Autodesk Inventor part; units mm, degrees
ref_plane "YZ Plane" through (0, 0, 0) normal (1, 0, 0) x (0, 1, 0)
ref_plane "XZ Plane" through (0, 0, 0) normal (0, 1, 0) x (-1, 0, 0)
ref_plane "XY Plane" through (0, 0, 0) normal (0, 0, 1) x (1, 0, 0)
sketch "Sketch1" plane through (0, 0, 0) normal (0, 1, 0) x (-1, 0, 0)
  line L0 (0, -15) -> (40, -15)
  line L1 (0, -54.7509) -> (0, -44.7509)
  line L2 (20, -23.5) -> (0, -23.5)
  line L3 (0, -23.5) -> (0, -15)
  circle A0 centre (5.2574, -19.75) radius 1.75
  line L4 (47.2, -27.5) -> (0, -54.7509)
  line L5 (0, -44.7509) -> (20, -33.2039)
  line L6 (20, -23.5) -> (20, -33.2039)
  line L7 (0, 15) -> (40, 15)
  line L8 (0, 54.7509) -> (0, 44.7509)
  line L9 (20, 23.5) -> (0, 23.5)
  line L10 (0, 23.5) -> (0, 15)
  circle A1 centre (5.2574, 19.75) radius 1.75
  line L11 (47.2, 27.5) -> (0, 54.7509)
  line L12 (0, 44.7509) -> (20, 33.2039)
  line L13 (20, 23.5) -> (20, 33.2039)
  line L14 (47.2, 27.5) -> (47.2, -27.5)
  line L15 (40, 15) -> (40, -15)
  line L16 (56.64, 0) -> (-9.44, 0)
  line L17 (0, -76.6513) -> (0, 76.6513)
  point P0 (0, 0)
  point P1 (0, 19.25)
  dimension "d3" = 15
  dimension "d6" = 5.2573
  dimension "d7" = 3.5
  dimension "d8" = 8.5
  dimension "d10" = 10
  dimension "d13" = 47.2
  dimension "d15" = 39.5
  dimension "d29" = 15
  dimension "d30" = 5.2573
  dimension "d31" = 40
  dimension "d32" = 19.75
  dimension "d33" = 8.5
  dimension "d34" = 20
  dimension "d35" = 20
  dimension "d37" = 60
  dimension "d38" = 60
  dimension "d39" = 55
  dimension "d40" = 27.5
  dimension "d41" = 10
  dimension "d68" = 21.2509
extrude "Extrusion1" add sketch "Sketch1" along normal blind 3 contours L0 L15 L16 L14 L4 L1 L5 L6 L2 L3 | L15 L7 L10 L9 L13 L12 L8 L11 L14 L16
sketch "Sketch2" plane through (0, 3, 0) normal (0, 1, 0) x (1, 0, 0)
  line L0 (-42.8964, 23) -> (-44.8964, 23)
  line L1 (-2.0164, 49.7415) -> (-1.0164, 48.0094)
  line L2 (-40.8535, 25.0094) -> (-41.8535, 26.7415)
  line L3 (-1.0164, -48.0094) -> (-2.0164, -49.7415)
  line L4 (-41.8535, -26.7415) -> (-40.8535, -25.0094)
  line L5 (-40.9205, -31.1255) -> (-39.2554, -28.2415)
  line L6 (-38.2554, -26.5094) -> (-36.5904, -23.6255)
  line L7 (-42.8964, -19.564) -> (-40.5928, -19.564)
  line L8 (-44.8964, -19.564) -> (-47.2, -19.564)
  line L9 (-47.2, 27.5) -> (-47.2, -27.5)
  line L10 (-47.2, -27.5) -> (-40.9205, -31.1255)
  line L11 (-47.2, -27.5) -> (0, -54.7509)
  line L12 (-4.6144, -48.2415) -> (-6.2795, -51.1255)
  line L13 (-3.6144, -46.5094) -> (-1.9494, -43.6255)
  line L14 (0, -44.7509) -> (-20, -33.2039)
  line L15 (-39.2554, 28.2415) -> (-40.9205, 31.1255)
  line L16 (-38.2554, 26.5094) -> (-36.5904, 23.6255)
  line L17 (-3.6144, 46.5094) -> (-1.9494, 43.6255)
  line L18 (-4.6144, 48.2415) -> (-6.2795, 51.1255)
  line L19 (-38.2554, -26.5094) -> (-40.8535, -25.0094)
  line L20 (-41.8535, -26.7415) -> (-39.2554, -28.2415)
  line L21 (-42.8964, -23) -> (-42.8964, -19.564)
  line L22 (-4.6144, -48.2415) -> (-2.0164, -49.7415)
  line L23 (-3.6144, -46.5094) -> (-1.0164, -48.0094)
  line L24 (-6.2795, -51.1255) -> (0, -54.7509)
  line L25 (0, -54.7509) -> (0, -44.7509)
  line L26 (0, -44.7509) -> (-1.9494, -43.6255)
  line L27 (-40.8535, 25.0094) -> (-38.2554, 26.5094)
  line L28 (-41.8535, 26.7415) -> (-39.2554, 28.2415)
  line L29 (-3.6144, 46.5094) -> (-1.0164, 48.0094)
  line L30 (-4.6144, 48.2415) -> (-2.0164, 49.7415)
  line L31 (-1.9494, 43.6255) -> (0, 44.7509)
  line L32 (0, 54.7509) -> (-6.2795, 51.1255)
  line L33 (0, 44.7509) -> (0, 54.7509)
  line L34 (-42.8964, 23) -> (-42.8964, 19.564)
  line L35 (-42.8964, 19.564) -> (-40.5928, 19.564)
  line L36 (-44.8964, 19.564) -> (-47.2, 19.564)
  line L37 (-47.2, 19.564) -> (-47.2, 27.5)
  line L38 (-47.2, 27.5) -> (-40.9205, 31.1255)
  line L39 (0, 54.7509) -> (-47.2, 27.5)
  line L40 (-20, 33.2039) -> (0, 44.7509)
  line L41 (-44.8964, -19.564) -> (-44.8964, -23)
  line L42 (-44.8964, -23) -> (-42.8964, -23)
  line L43 (-36.5904, 23.6255) -> (-40.5928, 21.3147)
  line L44 (-36.5904, -23.6255) -> (-40.5928, -21.3147)
  line L45 (-40.5928, -21.3147) -> (-40.5928, -19.564)
  line L46 (-40.5928, 19.564) -> (-40.5928, 21.3147)
  line L47 (-47.2, -27.5) -> (-47.2, -19.564)
  line L48 (-44.8964, 19.564) -> (-44.8964, 23)
  point P0 (0, 0)
  dimension "d20" = 2
  dimension "d21" = 46
  dimension "d25" = 2
  dimension "d44" = 3.3301
  dimension "d45" = 3.3301
  dimension "d46" = 46
  dimension "d47" = 3
  dimension "d48" = 3
  dimension "d49" = 7.2509
  dimension "d50" = 7.2509
  dimension "d53" = 3.3301
  dimension "d54" = 3.3301
  dimension "d55" = 3
  dimension "d56" = 3
  dimension "d57" = 7.2509
  dimension "d58" = 7.2509
  dimension "d59" = 2
  dimension "d61" = 2.3036
  dimension "d62" = 2.3036
  dimension "d63" = 2.3036
  dimension "d64" = 2.3036
  dimension "d72" = 46
  dimension "d73" = 2
  dimension "d74" = 2
  dimension "d75" = 3.3301
  dimension "d76" = 3.3301
  dimension "d77" = 7.936
  dimension "d78" = 7.936
extrude "Extrusion2" add sketch "Sketch2" along normal blind 3
fillet "Fillet1" radius 2 16 edges at (-47.2, 3, -27.5) (-47.2, 3, 27.5) (0, 3, 54.7509) (0, 3, 44.7509) (0, 1.5, -15) (0, 1.5, 23.5) (0, 1.5, 15) (0, 1.5, -23.5) (0, 3, -44.7509) (0, 3, -54.7509) (-20, 1.5, -23.5) (-20, 1.5, -33.2039) (-20, 1.5, 33.2039) (-20, 1.5, 23.5) (-40, 1.5, 15) (-40, 1.5, -15)
equation "\"d32\" = 0.5 * d15"
equation "\"d33\" = d8"
equation "\"d35\" = d34"
properties part number "walle"
Input: part model. Units: mm. Frame: model coordinates. A direction names the side the tool comes from. Give positions to 0.01 mm unless a question says otherwise; leave off trailing zeros. Order: outer loops, then holes, each group sorted by start corner. A loop starts at its lowest first (then second) coordinate and runs counter-clockwise, first axis right, second up.
1. Mould query, pull axis Z, two halves, no side actions, for faces 1 (the flat face through (-2, 6, -50)), 2 (the flat face through (-40.1, 4.479, 29.704)), 3 (the flat face through (-38.56, 4.48, -22.49)), 4 (the flat face through (-40.076, 4.479, -29.663)). Classes: released by +Z, released by -Z, zero draft, split by the parting line, or undercut.
Derived:
face 1: zero draft
face 2: released by +Z
face 3: undercut
face 4: released by -Z
2. Section C-C on x = -23. Return the cut outline in (y, z).
Derived:
outline: (0, -41.47) - (3, -41.47) - (3, -15) - (0, -15) - close; (0, 15) - (3, 15) - (3, 41.47) - (0, 41.47) - close
3. Material intervals for L1, parallel to Y at x = -11.5, z = -39; L2, parallel to Z at x = -9, y = 2.85; L3, parallel to Z at x = -11, y = 2, sorted ascending.
Derived:
L1: y = 0 to 3
L2: z = -49.55 to -39.55, -23.5 to -15, 15 to 23.5, 39.55 to 49.55
L3: z = -48.4 to -38.4, -23.5 to -15, 15 to 23.5, 38.4 to 48.4
4. Reachability of faces 5 (the flat face through (-5.435, 4.479, 49.663)), 6 (the flat face through (-20, 1, -15)), 7 (the flat face through (-40.573, 4.479, -27.481)) from +Z, -Z, +X, -X, +Y, -Y: full face, straight path, thin tool, end or side. Return the list, or none.
Derived:
face 5: -X, +Y
face 6: +X, +Y, -Y
face 7: +X, +Y
5. Pin query (flat end, axial travel): pin 1 (2.5 mm diameter, centred on x = -12, y = 1.5, fed in from +Z); pin 2 (1.5 mm diameter, centred on y = 1.5, z = -1.5, fed in from +X); pin 3 (2.5 mm diameter, centred on x = -6.5, y = 1, fed in from -Z); pin 4 (3 mm diameter, centred on x = -5.26, z = -19.75, fed in from +Y). Return the tip coordinate at first contact, or that it passes through.
Derived:
pin 1: stops at z = 48.54
pin 2: stops at x = -40
pin 3: stops at z = -51.72
pin 4: passes through
6. Section B-B on x = -11. Return the cut outline in (y, z).
Derived:
outline: (0, -48.4) - (3, -48.4) - (3, -38.4) - (0, -38.4) - close; (0, -23.5) - (3, -23.5) - (3, -15) - (0, -15) - close; (0, 15) - (3, 15) - (3, 23.5) - (0, 23.5) - close; (0, 38.4) - (3, 38.4) - (3, 48.4) - (0, 48.4) - close
7. Section A-A on y = 1.15. Give the number of separate pieces and of enclosed holes in the cut face, and give its area (3 significant figures).
Derived:
separate pieces: 1
enclosed holes: 2
area: 2,040 mm2
